from build123d import *

# Parameters (mm, degrees)
BASE_FLANGE1_DEPTH = 10
CUT_EXTRUDE1_DEPTH = 464.357313528
CUT_EXTRUDE2_DEPTH = 464.357313528
FILLET1_R          = 10
FILLET2_R          = 5
SKETCH8_R          = 7.5
CUT_EXTRUDE3_DEPTH = 460.635608137
SKETCH9_W          = 52
SKETCH9_H          = 12
CUT_EXTRUDE4_DEPTH = 460.635608137
SKETCH10_R         = 2
CUT_EXTRUDE5_DEPTH = 460.635608137


# Sheet-metal steps are written as plain solids
with BuildPart() as part:
    # Sketch1 → Base-Flange1 (new body)
    with BuildSketch(Plane(origin=(0, 0, 0), x_dir=(0, 0, -1), z_dir=(1, 0, 0))):
        Polygon((0, 0), (200, 315), (200, 390), (-250, 85), (-250, 0), align=None)
    extrude(amount=-BASE_FLANGE1_DEPTH)

    # Sketch6 → Cut-Extrude1 (cut, through all)
    with BuildSketch(Plane(origin=(0, 0, 0), x_dir=(0, 0, -1), z_dir=(1, 0, 0))):
        with BuildLine():
            Line((-212.5, 36), (-187.5, 36))
            ThreePointArc((-187.5, 36), (-181.5, 30), (-187.5, 24))
            Line((-187.5, 24), (-212.5, 24))
            ThreePointArc((-212.5, 24), (-218.5, 30), (-212.5, 36))
        make_face()
        with BuildLine():
            Line((-37.5, 36), (-62.5, 36))
            ThreePointArc((-62.5, 36), (-68.5, 30), (-62.5, 24))
            Line((-62.5, 24), (-37.5, 24))
            ThreePointArc((-37.5, 24), (-31.5, 30), (-37.5, 36))
        make_face()
    extrude(amount=-CUT_EXTRUDE1_DEPTH, mode=Mode.SUBTRACT)

    # Sketch7 → Cut-Extrude2 (cut, through all)
    with BuildSketch(Plane(origin=(0, 0, 0), x_dir=(0, 0, -1), z_dir=(1, 0, 0))):
        Polygon((80, 248.264209845), (-138.750473541, 100), (4.265291407, 100), (80, 219.282166034), align=None)
    extrude(amount=-CUT_EXTRUDE2_DEPTH, mode=Mode.SUBTRACT)

    # Fillet1
    fillet1_edges = [part.edges().sort_by_distance(p)[0] for p in [
        (-5, 219.282166034, -80),
        (-5, 100, -4.265291407),
    ]]
    fillet(fillet1_edges, radius=FILLET1_R)

    # Fillet2
    fillet2_edges = [part.edges().sort_by_distance(p)[0] for p in [
        (-5, 248.264209845, -80),
        (-5, 100, 138.750473541),
        (-5, 0, 250),
        (-5, 85, 250),
        (-5, 390, -200),
        (-5, 315, -200),
        (-5, 0, 0),
    ]]
    fillet(fillet2_edges, radius=FILLET2_R)

    # Sketch8 → Cut-Extrude3 (cut, through all)
    with BuildSketch(Plane(origin=(0, 0, 0), x_dir=(0, 0, -1), z_dir=(1, 0, 0))):
        with Locations((170, 330)):
            Circle(SKETCH8_R)
    extrude(amount=-CUT_EXTRUDE3_DEPTH, mode=Mode.SUBTRACT)

    # Sketch9 → Cut-Extrude4 (cut, through all)
    with BuildSketch(Plane(origin=(0, 0, 0), x_dir=(0, 0, -1), z_dir=(1, 0, 0))):
        with Locations((-125, 76)):
            Rectangle(SKETCH9_W, SKETCH9_H)
    extrude(amount=-CUT_EXTRUDE4_DEPTH, mode=Mode.SUBTRACT)

    # Sketch10 → Cut-Extrude5 (cut, through all)
    with BuildSketch(Plane(origin=(0, 0, 0), x_dir=(0, 0, -1), z_dir=(1, 0, 0))):
        with Locations((-150.292893219, 70.707106781)):
            Circle(SKETCH10_R)
        with Locations((-150.292893219, 81.292893219)):
            Circle(SKETCH10_R)
        with Locations((-99.707106781, 81.292893219)):
            Circle(SKETCH10_R)
        with Locations((-99.707106781, 70.707106781)):
            Circle(SKETCH10_R)
    extrude(amount=-CUT_EXTRUDE5_DEPTH, mode=Mode.SUBTRACT)


solid = part.part
Design review of the part built by this model. Coordinates are the model's own, in mm. A direction names the side the tool comes from. Round coordinates to 2 decimals unless told otherwise and drop trailing zeros. Order: outer loops, then holes, each group sorted by start corner. A loop starts at its lowest first (then second) coordinate and runs counter-clockwise, first axis right, second up.
1) For L1, parallel to Y at x = -6, z = 103; L2, parallel to Z at x = -3, y = 26; L3, parallel to Y at x = -6.5, z = 42.5, list the stretches that pass through material, from the lowest coordinate up.
The answers:
L1: y = 0 to 70, 82 to 100, 124.23 to 184.63
L2: z = -16.51 to 33.03, 66.97 to 183.03, 216.97 to 250
L3: y = 0 to 24, 36 to 100, 165.24 to 225.64
2) Consider section C-C (x = -3.5). Count the separate pieces of the cut face and the enclosed holes in it, plus the area to 3 significant figures.
The answers:
separate pieces: 1
enclosed holes: 5
area: 62,100 mm2
3) Consider section D-D (y = 330). State the section outline as (x, z) points, plus the area to 3 significant figures.
The answers:
outline: (-10, -200) - (0, -200) - (0, -177.5) - (-10, -177.5) - close; (-10, -162.5) - (0, -162.5) - (0, -111.48) - (-10, -111.48) - close
area: 735 mm2
4) Consider section B-B (y = 30). State the section outline as (x, z) points, plus the area to 3 significant figures.
The answers:
outline: (-10, -19.05) - (0, -19.05) - (0, 31.5) - (-10, 31.5) - close; (-10, 68.5) - (0, 68.5) - (0, 181.5) - (-10, 181.5) - close; (-10, 218.5) - (0, 218.5) - (0, 250) - (-10, 250) - close
area: 1,950 mm2
5) Machinability: for faces 4 (the flat face through (-4.93, 237.686, 24.725)), 5 (the cylindrical face through (-5.1, 103.4, 127.2)), which of the approach directions +Z, -Z, +X, -X, +Y, -Y give a long, thin tool a straight path to every point of the face, cutting with its end or side? Answer none if there is none.
The answers:
face 4: +Z, +X, -X, +Y
face 5: +X, -X
6) Draft analysis for pull direction Y (two halves, no side actions). For faces 1 (the flat face through (-4.93, 159.95, -42.33)), 2 (the flat face through (-5, 44, 250)), 3 (the flat face through (-5, 0, 126)), state which applies: released by +Y, released by -Y, zero draft, split by the parting line, or undercut.
The answers:
face 1: undercut
face 2: zero draft
face 3: released by -Y
7) Consider section A-A (z = -170). State the section outline as (x, y) points, plus the area to 3 significant figures.
The answers:
outline: (-10, 267.75) - (0, 267.75) - (0, 322.5) - (-10, 322.5) - close; (-10, 337.5) - (0, 337.5) - (0, 369.67) - (-10, 369.67) - close
area: 869 mm2
8) Clearance check with flat-ended pins moving along their axes: pin 1 Ø5 at (x, z) = (-6.5, 56) entering from +Y; pin 2 Ø3.5 at (y, z) = (81.29, 150.29) entering from +X; pin 3 Ø5 at (x, z) = (-5, -85) entering from +Y; pin 4 Ø3 at (x, y) = (-4.5, 252) entering from -Z. State where each tip first meets the part, or that it passes through.
The answers:
pin 1: stops at y = 218.18
pin 2: passes through
pin 3: stops at y = 313.75
pin 4: stops at z = -160.95
